Part model, mm, in its own coordinate system. Give positions to 0.01 mm unless a question says otherwise; leave off trailing zeros. Order: outer loops, then holes, each group sorted by start corner. A loop starts at its lowest first (then second) coordinate and runs counter-clockwise, first axis right, second up. Notation, with made-up numbers: (-29.75, -6) -> (14.25, -6) arc R29 cw to (14.25, 22) -> close; hole circle Ø10 at (16.5, 41.5). An arc over 180 degrees is marked (long way). Write item = value, one per line. Start each with the question number.
(1) Saw through at A-A, the plane z = 0. List the corners of the cut face in (x, y), then the cut area to 3 significant figures.
(2) Saw through at D-D, the plane y = 5.5. List the corners of the cut face in (x, z), then the cut area to 3 significant figures.
(3) Saw through at C-C, the plane x = 1.2. List the corners of the cut face in (y, z), then the cut area to 3 significant figures.
(4) Probe line 1 along Z through (x, y) = (1.4, -9.5); line 2 along Z through (x, y) = (1.5, -10); line 3 along Z through (x, y) = (1.5, 5). List the from-to ranges inside material, lowest first. Write a range as from..to.
(5) Saw through at B-B, the plane z = -16. List the corners of the cut face in (x, y).
Autodesk Inventor part; units mm, degrees
ref_plane "YZ Plane" through (0, 0, 0) normal (1, 0, 0) x (0, 1, 0)
ref_plane "XZ Plane" through (0, 0, 0) normal (0, 1, 0) x (-1, 0, 0)
ref_plane "XY Plane" through (0, 0, 0) normal (0, 0, 1) x (1, 0, 0)
sketch "Sketch1" plane through (0, 0, 0) normal (1, 0, 0) x (0, 1, 0)
  line L0 (-15.5, 21) -> (15.5, 21)
  line L1 (15.5, 21) -> (15.5, -21)
  line L2 (15.5, -21) -> (-15.5, -21)
  line L3 (-15.5, -21) -> (-15.5, 21)
  line L4 (-15.5, 21) -> (15.5, -21) construction
  line L5 (15.5, 21) -> (-15.5, -21) construction
  circle A0 centre (5.5, 16) radius 1.6
  circle A1 centre (5.5, -16) radius 1.6
  circle A2 centre (-9.5, -16) radius 1.6
  circle A3 centre (-9.5, 16) radius 1.6
  circle A4 centre (0, 0) radius 6
  point P0 (5.5, -16)
  point P1 (-9.5, -16)
  dimension "d0" = 42
  dimension "d1" = 31
  dimension "d2" = 5
  dimension "d3" = 10
  dimension "d5" = 15
  dimension "d6" = 5
  dimension "d7" = 3.2
  dimension "d8" = 3.2
  dimension "d9" = 3.2
  dimension "d10" = 3.2
  dimension "d11" = 12
extrude "Extrusion1" add sketch "Sketch1" along normal blind 2
fillet "Fillet1" radius 2 4 edges at (1, 15.5, 21) (1, -15.5, 21) (1, -15.5, -21) (1, 15.5, -21)
properties part number "2mm_double_for_pulley" material "アルミニウム 6061"
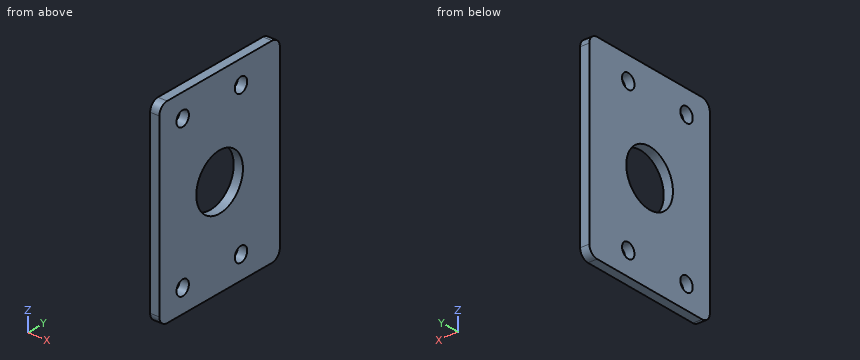
Results list:
q1.outline = (0, -15.5) -> (2, -15.5) -> (2, -6) -> (0, -6) -> close; (0, 6) -> (2, 6) -> (2, 15.5) -> (0, 15.5) -> close
q1.area = 38.0 mm^2
q2.outline = (0, -21) -> (2, -21) -> (2, -17.6) -> (0, -17.6) -> close; (0, -14.4) -> (2, -14.4) -> (2, -2.4) -> (0, -2.4) -> close; (0, 2.4) -> (2, 2.4) -> (2, 14.4) -> (0, 14.4) -> close; (0, 17.6) -> (2, 17.6) -> (2, 21) -> (0, 21) -> close
q2.area = 61.6 mm^2
q3.outline = (-15.5, -19) arc R2 ccw to (-13.5, -21) -> (13.5, -21) arc R2 ccw to (15.5, -19) -> (15.5, 19) arc R2 ccw to (13.5, 21) -> (-13.5, 21) arc R2 ccw to (-15.5, 19) -> close; hole circle Ø3.2 at (-9.5, -16); hole circle Ø3.2 at (-9.5, 16); hole circle Ø12 at (0, 0); hole circle Ø3.2 at (5.5, -16); hole circle Ø3.2 at (5.5, 16)
q3.area = 1,150 mm^2
q4.line_1 = -21..-17.6, -14.4..14.4, 17.6..21
q4.line_2 = -21..-17.52, -14.48..14.48, 17.52..21
q4.line_3 = -21..-17.52, -14.48..-3.32, 3.32..14.48, 17.52..21
q5.outline = (0, -15.5) -> (2, -15.5) -> (2, -11.1) -> (0, -11.1) -> close; (0, -7.9) -> (2, -7.9) -> (2, 3.9) -> (0, 3.9) -> close; (0, 7.1) -> (2, 7.1) -> (2, 15.5) -> (0, 15.5) -> close
